For this review, take the finished solid that the model builds, in its own axes (mm). A direction names the side the tool comes from. Round coordinates to 2 decimals unless told otherwise and drop trailing zeros. Order: outer loops, then holes, each group sorted by start corner. A loop starts at its lowest first (then second) coordinate and runs counter-clockwise, first axis right, second up. Notation, with made-up numbers: (69, 0.25) -> (99, 0.25) arc R19 ccw to (99, 17.25) -> close; hole circle Ø7 at (83, 26). An arc over 180 degrees is marked (long way). Put each result on its own line as item: value. Start each with the question number.
```python
from build123d import *

# Parameters (mm, degrees)
SKETCH2_R           = 6.35
BOSS_EXTRUDE1_DEPTH = 10.922
SKETCH3_W           = 11.565028963
SKETCH3_H           = 5.944743938
CUT_EXTRUDE1_DEPTH  = 15.24
SKETCH4_R           = 1.5
CUT_EXTRUDE2_DEPTH  = 5.08
SKETCH6_R           = 2.05
CUT_EXTRUDE3_DEPTH  = 10.16
BOSS_EXTRUDE2_DEPTH = 34.798
SKETCH9_R           = 1.905
BOSS_EXTRUDE3_DEPTH = 7.62


with BuildPart() as part:
    # Sketch2 → Boss-Extrude1 (new body)
    with BuildSketch(Plane.XY):
        Circle(SKETCH2_R)
    extrude(amount=BOSS_EXTRUDE1_DEPTH)

    # Sketch3 → Cut-Extrude1 (cut)
    with BuildSketch(Plane.XY.offset(10.922)):
        with Locations((0.956423272, 7.099276819)):
            Rectangle(SKETCH3_W, SKETCH3_H)
    extrude(amount=-CUT_EXTRUDE1_DEPTH, mode=Mode.SUBTRACT)

    # Sketch4 → Cut-Extrude2 (cut)
    with BuildSketch(Plane(origin=(0, 4.12690485, 0), x_dir=(1, 0, 0), z_dir=(0, 1, 0))):
        with Locations(Location((0, -5.461, 0), (0, 0, 270))):
            Circle(SKETCH4_R)
    extrude(amount=-CUT_EXTRUDE2_DEPTH, mode=Mode.SUBTRACT)

    # Sketch6 → Cut-Extrude3 (cut)
    with BuildSketch(Plane.XY.offset(10.922)):
        Circle(SKETCH6_R)
    extrude(amount=-CUT_EXTRUDE3_DEPTH, mode=Mode.SUBTRACT)

    # Sketch8 → Boss-Extrude2 (add)
    with BuildSketch(Plane(origin=(0, 0, 0), x_dir=(-1, 0, 0), z_dir=(0, 0, -1))):
        Polygon((0, 4.064), (-3.519527241, -2.032), (3.519527241, -2.032), align=None)
    extrude(amount=BOSS_EXTRUDE2_DEPTH)

    # Sketch9 → Boss-Extrude3 (add)
    with BuildSketch(Plane(origin=(0, 0, -34.798), x_dir=(-1, 0, 0), z_dir=(0, 0, -1))):
        with Locations(Location((0, 0, 0), (0, 0, 180))):
            Circle(SKETCH9_R)
    extrude(amount=BOSS_EXTRUDE3_DEPTH)


solid = part.part
```
Item 1: Mouldability with a two-part tool opening along X and no side actions: class faces 1 (the face through (-0.91, 2.78, 4.27)), 2 (the face through (-0.203, -6.347, 5.385)), 3 (the face through (-1.784, 0.973, -17.155)), 4 (the face through (0, -2.032, -17)) as +X half, -X half, draft (parallel to the pull), parting line (faces both ways), or undercut.
Item 2: Tool access review of faces 5 (the face through (1.735, 1.059, -17.155)), 6 (the face through (0, 0, -42.418)), 7 (the face through (-0.25, -1.89, -38.55)), 8 (the face through (0, 0, 0.762)): name each direction out of +Z, -Z, +X, -X, +Y, -Y from which nothing blocks a thin tool from reaching the whole face with its end or side.
Item 3: Consider section B-B, the plane y = 0. Write out the cut boundary in (x, z) (3 decimals), plus the area to 3 significant figures.
Item 4: Insertion check: pin 1 Ø5 at (x, y) = (-4.5, 1.5) entering from -Z; pin 2 Ø2 at (x, z) = (0, -16.5) entering from -Y. Each pin has a flat end and moves straight along its axis. Give the tip position at first contact, or say it passes through.
Item 5: For L1, parallel to Z at x = 0, y = 3.5; L2, parallel to Z at x = 0.5, y = -0.5; L3, parallel to Z at x = -1.75, y = 2.5, list the stretches that pass through material, from the lowest coordinate up.
Item 6: Consider section D-D, the plane z = -31.5. Write out the cut boundary in (x, y).
Item 7: Consider section A-A, the plane z = 1.5. Write out the cut boundary in (x, y).
Item 8: Consider section C-C, the plane x = -3. Write out the cut boundary in (y, z).
Evaluation:
1. face 1: undercut
1. face 2: parting line
1. face 3: -X half
1. face 4: draft
2. face 5: -Z, +X, +Y
2. face 6: -Z, +X, -X, +Y, -Y
2. face 7: -Z
2. face 8: +Z
3. outline: (-6.35, 0) -> (-2.346, 0) -> (-2.346, -34.798) -> (-1.905, -34.798) -> (-1.905, -42.418) -> (1.905, -42.418) -> (1.905, -34.798) -> (2.346, -34.798) -> (2.346, 0) -> (6.35, 0) -> (6.35, 10.922) -> (2.05, 10.922) -> (2.05, 0.762) -> (-2.05, 0.762) -> (-2.05, 10.922) -> (-6.35, 10.922) -> close
3. area: 289 mm^2
4. pin 1: stops at z = 0
4. pin 2: stops at y = -2.03
5. L1: z = -34.8 to 3.96, 6.96 to 10.92
5. L2: z = -42.42 to 0.76
5. L3: z = 0 to 10.92
6. outline: (-3.52, -2.03) -> (3.52, -2.03) -> (0, 4.06) -> close
7. outline: (-4.83, 4.13) arc R6.35 ccw (long way) to (4.83, 4.13) -> close; hole circle Ø4.1 at (0, 0)
8. outline: (-5.6, 0) -> (-2.03, 0) -> (-2.03, -34.8) -> (-1.13, -34.8) -> (-1.13, 0) -> (4.13, 0) -> (4.13, 10.92) -> (-5.6, 10.92) -> close
